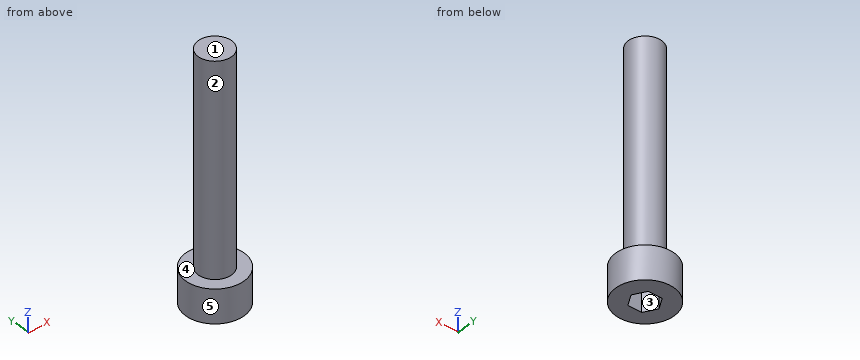
Solid Edge part; units mm, degrees
sketch "Sketch1" plane through (0, 0, 0) normal (0, 0, 1) x (1, 0, 0)
  circle A0 centre (0, 0) radius 3.5
extrude "Protrusion1" add sketch "Sketch1" along normal blind 4
sketch "Sketch2" plane through (0, 0, 0) normal (0, 0, -1) x (1, 0, 0)
  line L0 (0.85, 1.4722) -> (1.7, 0)
  line L1 (1.7, 0) -> (0.85, -1.4722)
  line L2 (0.85, -1.4722) -> (-0.85, -1.4722)
  line L3 (-0.85, -1.4722) -> (-1.7, 0)
  line L4 (-1.7, 0) -> (-0.85, 1.4722)
  line L5 (-0.85, 1.4722) -> (0.85, 1.4722)
extrude "ExtrudedCutout_1" cut sketch "Sketch2" against normal blind 2.4
sketch "Sketch3" plane through (0, 0, 4) normal (0, 0, 1) x (-1, 0, 0)
  circle A0 centre (0, 0) radius 2
extrude "ExtrudedProtrusion_2" add sketch "Sketch3" along normal blind 25
cosmetic_thread "Thread_1" thread depth 20
Could you check a few things on this model? Use its own coordinates, in mm. Face numbers are marked on the shaded views. A direction names the side the tool comes from. Give positions to 0.01 mm unless a question says otherwise; leave off trailing zeros. Order: outer loops, then holes, each group sorted by start corner. A loop starts at its lowest first (then second) coordinate and runs counter-clockwise, first axis right, second up. Notation, with made-up numbers: (-28.75, -29) - (9.25, -29) arc R31 ccw to (9.25, 2) - close; hole circle Ø7 at (48, 34). An arc over 180 degrees is marked (long way). Return JSON: item names as keys, results as strings. Group by question number.
Q1. Please list where these lines run through material, in increasing order: line 1 along Z through (x, y) = (1.75, 1.75); line 2 along X through (y, z) = (0, 14.25); line 3 along Z through (x, y) = (-0.5, 0.25). Write a range as [from, to].
Q2. Thinking about a two-plate mould opening in Y: for the marked faces 3, 4 and 5, which applies, pulls with the +Y half, pulls with the -Y half, needs draft (parallel to the pull), parting line crosses it, or undercut?
Q3. Will these pins go through, and if not, where does the flat tip stop? pin 1 Ø3 at (y, z) = (-2, 9) entering from +X; pin 2 Ø1.5 at (x, y) = (-0.5, -0.5) entering from -Z; pin 3 Ø3 at (x, z) = (1.5, 22) entering from -Y.
Q4. Suppose I cut it at D-D, the plane x = -3. Please give me the cut outline in (y, z), and give its area (3 significant figures).
Q5. Suppose I cut it at A-A, the plane x = 0. Please give me the cut outline in (y, z), and give its area (3 significant figures).
Q6. Suppose I cut it at B-B, the plane y = -0.25. Please give me the cut outline in (x, z), and give its area (3 significant figures).
Q7. Which directions (+Z, -Z, +X, -X, +Y, -Y) give clear straight access to the entire face, cutting with the end or side of a thin tool? Please do the marked faces 1 and 2.
Q8. Suppose I cut it at C-C, the plane z = 27.25. Please give me the cut outline in (x, y).
Resolved:
{
 "1": {"line 1": "z = [0, 4]", "line 2": "x = [-2, 2]", "line 3": "z = [2.4, 29]"},
 "2": {"face 3": "undercut", "face 4": "needs draft", "face 5": "parting line crosses it"},
 "3": {"pin 1": "stops at x = 1.94", "pin 2": "stops at z = 2.4", "pin 3": "stops at y = -2"},
 "4": {"outline": "(-1.8, 0) - (1.8, 0) - (1.8, 4) - (-1.8, 4) - close", "area": "14.4 mm2"},
 "5": {"outline": "(-3.5, 0) - (-1.47, 0) - (-1.47, 2.4) - (1.47, 2.4) - (1.47, 0) - (3.5, 0) - (3.5, 4) - (2, 4) - (2, 29) - (-2, 29) - (-2, 4) - (-3.5, 4) - close", "area": "121 mm2"},
 "6": {"outline": "(-3.49, 0) - (-1.56, 0) - (-1.56, 2.4) - (1.56, 2.4) - (1.56, 0) - (3.49, 0) - (3.49, 4) - (1.98, 4) - (1.98, 29) - (-1.98, 29) - (-1.98, 4) - (-3.49, 4) - close", "area": "120 mm2"},
 "7": {"face 1": "+Z, +X, -X, +Y, -Y", "face 2": "+Z"},
 "8": {"outline": "circle Ø4 at (0, 0)"}
}
